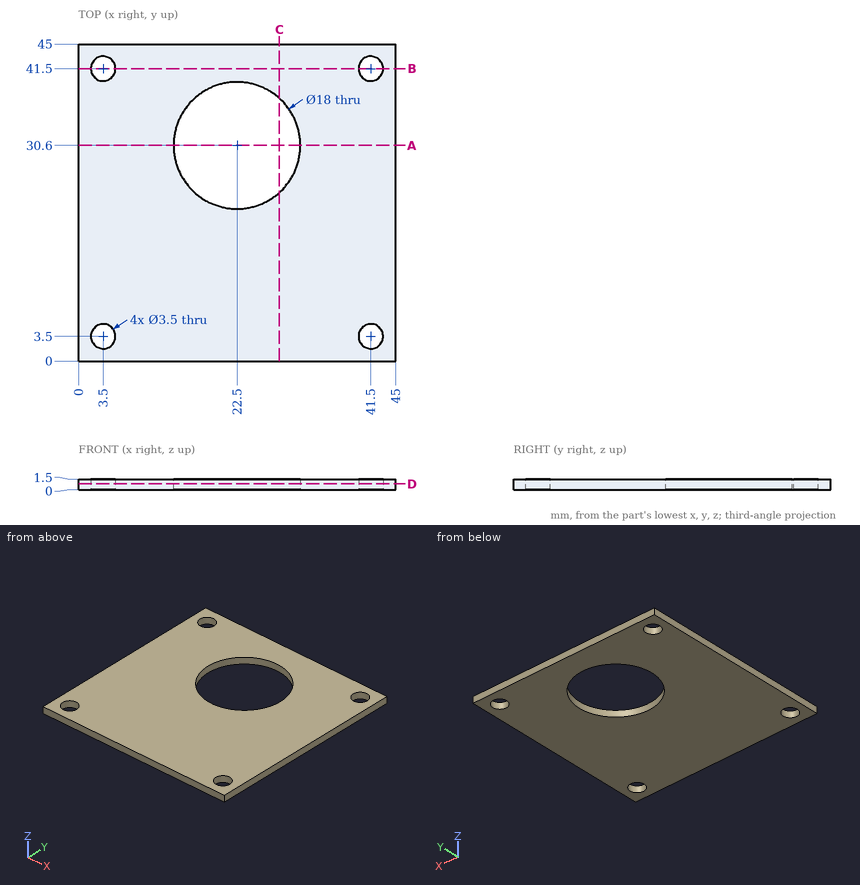
Design review of the part shown in the three views and the two pictorial views. Dimensions are in mm from the part's minimum x, y and z. Round coordinates to 2 decimals unless told otherwise and drop trailing zeros. Loops run counter-clockwise (first coordinate to the right, second up) from the corner with the lowest first, then second, coordinate; pieces in that order, holes last. Notation, with made-up numbers: M 17.5,41 L 39.5,41 A20 cw 39.5,56 Z; hole C 60,37.5 d10. An arc over 180 degrees is marked long. Write item = value, one per line.
Item 1: For line 1 (Y direction, x = 3.5, z = 0.5); line 2 (Y direction, x = 22.5, z = 1.1); line 3 (X direction, y = 41, z = 0.5), list the stretches that pass through material, from the lowest coordinate up. Write a range as [from, to].
Return value:
line_1 = [0, 1.75], [5.25, 39.75], [43.25, 45]
line_2 = [0, 21.6], [39.6, 45]
line_3 = [0, 1.82], [5.18, 39.82], [43.18, 45]
Item 2: Take a section at A-A on y = 30.6. Write out the cut boundary in (x, z), then the cut area to 3 significant figures.
Return value:
outline = M 0,0 L 13.5,0 L 13.5,1.5 L 0,1.5 Z; M 31.5,0 L 45,0 L 45,1.5 L 31.5,1.5 Z
area = 40.5 mm2
Item 3: Take a section at C-C on x = 28.5. Write out the cut boundary in (y, z), then the cut area to 3 significant figures.
Return value:
outline = M 0,0 L 23.89,0 L 23.89,1.5 L 0,1.5 Z; M 37.31,0 L 45,0 L 45,1.5 L 37.31,1.5 Z
area = 47.4 mm2
Item 4: Take a section at B-B on y = 41.5. Write out the cut boundary in (x, z).
Return value:
outline = M 0,0 L 1.75,0 L 1.75,1.5 L 0,1.5 Z; M 5.25,0 L 39.75,0 L 39.75,1.5 L 5.25,1.5 Z; M 43.25,0 L 45,0 L 45,1.5 L 43.25,1.5 Z
Item 5: Take a section at D-D on z = 0.8. Write out the cut boundary in (x, y), then the cut area to 3 significant figures.
Return value:
outline = M 0,0 L 45,0 L 45,45 L 0,45 Z; hole C 3.5,3.5 d3.5; hole C 3.5,41.5 d3.5; hole C 22.5,30.6 d18; hole C 41.5,3.5 d3.5; hole C 41.5,41.5 d3.5
area = 1,730 mm2
